from build123d import *

# Parameters (mm, degrees)
BOSS_EXTRUDE1_DEPTH = 3
SKETCH2_W           = 3.4
SKETCH2_H           = 144.72
BOSS_EXTRUDE2_DEPTH = 31.5
SKETCH3_R           = 1.5
CUT_EXTRUDE1_DEPTH  = 40
FILLET1_R           = 2
FILLET2_R           = 2


with BuildPart() as part:
    # Sketch1 → Boss-Extrude1 (new body)
    with BuildSketch(Plane(origin=(0, 0, 0), x_dir=(1, 0, 0), z_dir=(0, 1, 0))):
        Polygon((-79.175996169, 45), (-79.175996169, -45), (-4, -72.36), (0, -72.36), (0, 72.36), (-4, 72.36), align=None)
    extrude(amount=BOSS_EXTRUDE1_DEPTH)

    # Sketch2 → Boss-Extrude2 (add)
    with BuildSketch(Plane.XZ):
        with Locations((-1.7, 0)):
            Rectangle(SKETCH2_W, SKETCH2_H)
    extrude(amount=-BOSS_EXTRUDE2_DEPTH)

    # Sketch3 → Cut-Extrude1 (cut)
    with BuildSketch(Plane(origin=(0, 3, 0), x_dir=(1, 0, 0), z_dir=(0, 1, 0))):
        with Locations(Location((-75.899387992, -42.705694255, 0), (0, 0, 270))):
            Circle(SKETCH3_R)
        with Locations(Location((-75.899387992, 42.705694255, 0), (0, 0, 270))):
            Circle(SKETCH3_R)
    extrude(amount=-CUT_EXTRUDE1_DEPTH, mode=Mode.SUBTRACT)

    # Fillet1
    # the kernel refuses this fillet: 2 mm, written as the material it takes off along each edge
    with BuildSketch(Plane(origin=(-9, 0, -72.36), x_dir=(0, 0, 1), z_dir=(1, 0, 0)), Plane(origin=(5, 0, 72.36), x_dir=(0, 0, -1), z_dir=(-1, 0, 0))) as fillet1_piece_1:
        with BuildLine():
            CenterArc((FILLET1_R, -FILLET1_R), FILLET1_R, 90, 90)
            Line((0, -FILLET1_R), (0, 0))
            Line((0, 0), (FILLET1_R, 0))
        make_face()
    extrude(amount=14, mode=Mode.SUBTRACT)
    with BuildSketch(Plane(origin=(0, 0, 77.36), x_dir=(-1, 0, 0), z_dir=(0, 0, -1))) as fillet1_piece_2:
        with BuildLine():
            CenterArc((FILLET1_R, FILLET1_R), FILLET1_R, 180, 90)
            Line((0, FILLET1_R), (0, 0))
            Line((0, 0), (FILLET1_R, 0))
        make_face()
    extrude(amount=154.72, mode=Mode.SUBTRACT)
    with BuildSketch(Plane(origin=(-83.87449593, 0, 43.29), x_dir=(0, 1, 0), z_dir=(0.9396999521123751, 0, 0.34199999999999997)), Plane(origin=(0.698499761, 0, -74.07), x_dir=(0, 1, 0), z_dir=(-0.9396999521123751, 0, 0.34199999999999997))) as fillet1_piece_3:
        with BuildLine():
            CenterArc((FILLET1_R, -FILLET1_R), FILLET1_R, 90, 90)
            Line((0, -FILLET1_R), (0, 0))
            Line((0, 0), (FILLET1_R, 0))
        make_face()
    extrude(amount=90, mode=Mode.SUBTRACT)
    with BuildSketch(Plane(origin=(-79.175996169, 0, -50), x_dir=(0, 1, 0), z_dir=(0, 0, 1))) as fillet1_piece_4:
        with BuildLine():
            CenterArc((FILLET1_R, -FILLET1_R), FILLET1_R, 90, 90)
            Line((0, -FILLET1_R), (0, 0))
            Line((0, 0), (FILLET1_R, 0))
        make_face()
    extrude(amount=100, mode=Mode.SUBTRACT)

    # Fillet2
    # the kernel refuses this fillet: 2 mm, written as the material it takes off along each edge
    with BuildSketch(Plane(origin=(-2, 2, -70.36), x_dir=(1, 0, 0), z_dir=(0, 0, -1))) as fillet2_piece_1_section:
        Polygon((0, 0), (FILLET2_R, 0), (FILLET2_R, FILLET2_R), (0, FILLET2_R), align=None)
    fillet2_piece_1 = extrude(amount=FILLET2_R, mode=Mode.PRIVATE)
    fillet2_piece_1 = fillet2_piece_1 - Plane(origin=(-2, 2, -70.36), x_dir=(-0.7071067811865475, 0.7071067811865475, 0), z_dir=(0, 0, -1)) * Sphere(FILLET2_R, mode=Mode.PRIVATE)
    add(fillet2_piece_1, mode=Mode.SUBTRACT)
    with BuildSketch(Plane(origin=(-2, 2, 70.36), x_dir=(1, 0, 0), z_dir=(0, 0, 1))) as fillet2_piece_2_section:
        Polygon((0, 0), (FILLET2_R, 0), (FILLET2_R, -FILLET2_R), (0, -FILLET2_R), align=None)
    fillet2_piece_2 = extrude(amount=FILLET2_R, mode=Mode.PRIVATE)
    fillet2_piece_2 = fillet2_piece_2 - Plane(origin=(-2, 2, 70.36), x_dir=(-0.7071067811865475, 0.7071067811865475, 0), z_dir=(0, 0, 1)) * Sphere(FILLET2_R, mode=Mode.PRIVATE)
    add(fillet2_piece_2, mode=Mode.SUBTRACT)
    with BuildSketch(Plane(origin=(0, 36.5, -72.36), x_dir=(-1, 0, 0), z_dir=(0, -1, 0)), Plane(origin=(0, 2, 72.36), x_dir=(-1, 0, 0), z_dir=(0, 1, 0))) as fillet2_piece_3:
        with BuildLine():
            CenterArc((FILLET2_R, -FILLET2_R), FILLET2_R, 90, 90)
            Line((0, -FILLET2_R), (0, 0))
            Line((0, 0), (FILLET2_R, 0))
        make_face()
    extrude(amount=34.5, mode=Mode.SUBTRACT)


solid = part.part
Source: CAD feature listing. Evaluate the final solid. Frame: model axes, mm. A direction names the side the tool comes from. Coordinates: 2 decimals unless noted, no trailing zeros. Loops run counter-clockwise (first coordinate to the right, second up) from the corner with the lowest first, then second, coordinate; pieces in that order, holes last. Notation, with made-up numbers: (81, -5.5) - (91, -5.5) arc R17 ccw to (91, -1.5) - close; hole circle Ø10 at (3, 87.5). An arc over 180 degrees is marked (long way). Return JSON: item names as keys, results as strings.
Q1. Material intervals for line 1 along X through (y, z) = (6.5, -2.5); line 2 along Y through (x, z) = (-9, 40); line 3 along Z through (x, y) = (-29, 2), sorted ascending.
Results:
{"line 1": "-3.4 to 0", "line 2": "0 to 3", "line 3": "-63.26 to 63.26"}
Q2. Section A-A, the plane z = -2. Return loops of the section in (x, y).
Results:
{"outline": "(-79.18, 2) arc R2 ccw to (-77.18, 0) - (-2, 0) arc R2 ccw to (0, 2) - (0, 31.5) - (-3.4, 31.5) - (-3.4, 3) - (-79.18, 3) - close"}
Q3. Mould query, pull axis X, two halves, no side actions, for faces 3 (the flat face through (-41.062, 2.493, -58.872)), 4 (the flat face through (0, 17, 1)), 5 (the cylindrical face through (-76.812, 1.521, 41.515)). Classes: released by +X, released by -X, zero draft, split by the parting line, or undercut.
Results:
{"face 3": "released by -X", "face 4": "released by +X", "face 5": "undercut"}
Q4. Section B-B, the plane y = 16. Return loops of the section in (x, z), plus the area to 3 significant figures.
Results:
{"outline": "(-3.4, -72.36) - (-2, -72.36) arc R2 ccw to (0, -70.36) - (0, 70.36) arc R2 ccw to (-2, 72.36) - (-3.4, 72.36) - close", "area": "490 mm2"}
Q5. Access query for faces 1 (the flat face through (-42, 3, -1)), 2 (the cylindrical face through (-76.47, 1.52, -41.32)). Directions: +Z, -Z, +X, -X, +Y, -Y. A direction counts if a zero-diameter tool reaches every point of the face in a straight line with its end or side. Return the directions, or none.
Results:
{"face 1": "+Z, -Z, -X, +Y", "face 2": "+Y, -Y"}
Q6. Contact query for flat-ended pins moving along their axis: P1, Ø4, axis at y = 28, z = 41, coming from the -X side; P2, Ø12, axis at x = -32, z = 1.5, coming from the +Y side. Output: stop coordinate, or through.
Results:
{"P1": "x = -3.4", "P2": "y = 3"}
